Could you check a few things on this model? Use its own coordinates, in mm. A direction names the side the tool comes from. Coordinates: 2 decimals unless noted, no trailing zeros. Write each loop counter-clockwise with the first axis right and the second up, starting at its lowest first coordinate (ties: lowest second). Pieces come first, ordered by that corner, then holes.
```python
from build123d import *

# Parameters (mm, degrees)
SKETCH1_R           = 1.5
SKETCH1_R_2         = 4.25
SKETCH1_R_3         = 5
SKETCH1_R_4         = 1
BOSS_EXTRUDE2_DEPTH = 5
SKETCH2_W           = 0.5
SKETCH2_H           = 37
BOSS_EXTRUDE3_DEPTH = 5
CUT_EXTRUDE1_DEPTH  = 10
BOSS_EXTRUDE4_DEPTH = 5
SKETCH5_R           = 1.6
CUT_EXTRUDE2_DEPTH  = 10
BOSS_EXTRUDE5_DEPTH = 5
SKETCH7_R           = 1
BOSS_EXTRUDE6_DEPTH = 5


with BuildPart() as part:
    # Sketch1 → Boss-Extrude2 (new body)
    with BuildSketch(Plane.XY):
        with BuildLine():
            Line((45.25091594, -25.207708346), (50.00091594, -20.457708346))
            Line((50.00091594, -20.457708346), (50.00091594, 24.688738263))
            Line((50.00091594, 24.688738263), (45.147362549, 29.542291654))
            Line((45.147362549, 29.542291654), (26.35446933, 29.542291654))
            Line((26.35446933, 29.542291654), (21.25091594, 24.438738263))
            Line((21.25091594, 24.438738263), (21.25091594, 18.042291654))
            Line((21.25091594, 18.042291654), (20.408095363, 18.042291654))
            Line((20.408095363, 18.042291654), (16.70086026, 18.042291654))
            ThreePointArc((16.70086026, 18.042291654), (12.892426636, 17.542145454), (9.3422674, 16.075624987))
            ThreePointArc((9.3422674, 16.075624987), (2.182128173, 13.100539865), (-5.49908406, 12.043324729))
            Line((-5.49908406, 12.043324729), (-5.49908406, 12.039085999))
            ThreePointArc((-5.49908406, 12.039085999), (-15.49908406, 2.292291654), (-5.49908406, -7.454502691))
            Line((-5.49908406, -7.454502691), (-5.49908406, -7.458741422))
            ThreePointArc((-5.49908406, -7.458741422), (2.182128173, -8.515956557), (9.3422674, -11.491041679))
            ThreePointArc((9.3422674, -11.491041679), (12.892426636, -12.957562146), (16.70086026, -13.457708346))
            Line((16.70086026, -13.457708346), (20.408095363, -13.457708346))
            Line((20.408095363, -13.457708346), (21.25091594, -13.457708346))
            Line((21.25091594, -13.457708346), (21.25091594, -20.207708346))
            Line((21.25091594, -20.207708346), (26.25091594, -25.207708346))
            Line((26.25091594, -25.207708346), (45.25091594, -25.207708346))
        make_face()
        with Locations((46.75091594, -7.707708346)):
            Circle(SKETCH1_R, mode=Mode.SUBTRACT)
        with Locations((46.75091594, 12.292291654)):
            Circle(SKETCH1_R, mode=Mode.SUBTRACT)
        with Locations((33.50091594, 14.792291654)):
            Circle(SKETCH1_R_2, mode=Mode.SUBTRACT)
        with Locations((33.50091594, -10.207708346)):
            Circle(SKETCH1_R_2, mode=Mode.SUBTRACT)
        with Locations((19.25091594, 12.292291654)):
            Circle(SKETCH1_R, mode=Mode.SUBTRACT)
        with Locations((19.25091594, -7.707708346)):
            Circle(SKETCH1_R, mode=Mode.SUBTRACT)
        with Locations((-5.74908406, 2.292291654)):
            Circle(SKETCH1_R_3, mode=Mode.SUBTRACT)
        with Locations((1.25091594, 2.354746229)):
            Circle(SKETCH1_R_4, mode=Mode.SUBTRACT)
        with Locations((-5.686629485, -4.707708346)):
            Circle(SKETCH1_R_4, mode=Mode.SUBTRACT)
        with Locations((-12.74908406, 2.229837079)):
            Circle(SKETCH1_R_4, mode=Mode.SUBTRACT)
        with Locations((-5.811538636, 9.292291654)):
            Circle(SKETCH1_R_4, mode=Mode.SUBTRACT)
    extrude(amount=BOSS_EXTRUDE2_DEPTH)

    # Sketch2 → Boss-Extrude3 (add)
    with BuildSketch(Plane(origin=(0, 0, 0), x_dir=(-1, 0, 0), z_dir=(0, 0, -1))):
        Polygon((-26.25091594, -25.207708346), (-21.50091594, -25.207708346), (-21.50091594, -20.457708346), align=None)
        Polygon((-45.25091594, -25.207708346), (-45.50091594, -25.207708346), (-45.50091594, -24.957708346), align=None)
        Polygon((-45.50091594, 29.188738263), (-45.50091594, 29.792291654), (-21.50091594, 29.792291654), (-21.50091594, 24.688738263), (-26.35446933, 29.542291654), (-45.147362549, 29.542291654), align=None)
        with Locations((-50.25091594, 2.292291654)):
            Rectangle(SKETCH2_W, SKETCH2_H)
    extrude(amount=-BOSS_EXTRUDE3_DEPTH)

    # Sketch3 → Cut-Extrude1 (cut)
    with BuildSketch(Plane(origin=(0, 0, 0), x_dir=(-1, 0, 0), z_dir=(0, 0, -1))):
        Polygon((-50.00091594, -16.207708346), (-45.50091594, -16.207708346), (-45.50091594, -25.207708346), (-50.00091594, -20.457708346), align=None)
        Polygon((-50.50091594, 20.792291654), (-45.50091594, 20.792291654), (-45.50091594, 29.188738263), (-50.00091594, 24.688738263), align=None)
        Polygon((-21.50091594, -16.207708346), (-21.50091594, -20.457708346), (-21.25091594, -20.207708346), (-21.25091594, -16.207708346), align=None)
        Polygon((-21.50091594, 20.792291654), (-21.25091594, 20.792291654), (-21.25091594, 24.438738263), (-21.50091594, 24.688738263), align=None)
    extrude(amount=-CUT_EXTRUDE1_DEPTH, mode=Mode.SUBTRACT)

    # Sketch4 → Boss-Extrude4 (add)
    with BuildSketch(Plane(origin=(0, 0, 0), x_dir=(-1, 0, 0), z_dir=(0, 0, -1))):
        with BuildLine():
            Line((-21.25091594, 20.792291654), (-16.50091594, 20.792291654))
            Line((-16.50091594, 20.792291654), (-16.50091594, 18.040936414))
            ThreePointArc((-16.50091594, 18.040936414), (-16.600885803, 18.04195284), (-16.70086026, 18.042291654))
            Line((-16.70086026, 18.042291654), (-21.25091594, 18.042291654))
            Line((-21.25091594, 18.042291654), (-21.25091594, 20.792291654))
        make_face()
        with BuildLine():
            Line((-16.50091594, -13.456353106), (-16.50091594, -16.207708346))
            Line((-16.50091594, -16.207708346), (-21.25091594, -16.207708346))
            Line((-21.25091594, -16.207708346), (-21.25091594, -13.457708346))
            Line((-21.25091594, -13.457708346), (-16.70086026, -13.457708346))
            ThreePointArc((-16.70086026, -13.457708346), (-16.600885803, -13.457369532), (-16.50091594, -13.456353106))
        make_face()
    extrude(amount=-BOSS_EXTRUDE4_DEPTH)

    # Sketch5 → Cut-Extrude2 (cut)
    with BuildSketch(Plane.XY.offset(5)):
        with Locations((20.50091594, -7.707708346)):
            Circle(SKETCH5_R)
        with Locations((20.50091594, 12.292291654)):
            Circle(SKETCH5_R)
    extrude(amount=-CUT_EXTRUDE2_DEPTH, mode=Mode.SUBTRACT)

    # Sketch6 → Boss-Extrude5 (add)
    with BuildSketch(Plane.XY.offset(5)):
        with BuildLine():
            ThreePointArc((19.75191594, -6.293848735), (18.90091594, -7.707708346), (19.75191594, -9.121567957))
            ThreePointArc((19.75191594, -9.121567957), (17.75091594, -7.707708346), (19.75191594, -6.293848735))
        make_face()
        with BuildLine():
            ThreePointArc((19.75191594, 13.706151265), (18.90091594, 12.292291654), (19.75191594, 10.878432043))
            ThreePointArc((19.75191594, 10.878432043), (17.75091594, 12.292291654), (19.75191594, 13.706151265))
        make_face()
    extrude(amount=-BOSS_EXTRUDE5_DEPTH)

    # Sketch7 → Boss-Extrude6 (add)
    with BuildSketch(Plane(origin=(0, 0, 0), x_dir=(-1, 0, 0), z_dir=(0, 0, -1))):
        with Locations((-1.25091594, 2.354746229)):
            Circle(SKETCH7_R)
        with Locations((12.74908406, 2.229837079)):
            Circle(SKETCH7_R)
    extrude(amount=-BOSS_EXTRUDE6_DEPTH)


solid = part.part
```
1. For pin 1 (1 mm diameter, centred on x = 16.5, z = 1, fed in from +Y); pin 2 (7.5 mm diameter, centred on x = 33.5, y = -10.21, fed in from +Z); pin 3 (1 mm diameter, centred on y = 24, z = 0.5, fed in from -X); pin 4 (1.5 mm diameter, centred on x = 19, z = 2.5, fed in from -Y), each with a flat end and sliding along its axis, tell me the tip position at first contact or that it passes through.
Verdict:
pin 1: stops at y = 20.79
pin 2: passes through
pin 3: stops at x = 21.5
pin 4: stops at y = -16.21
2. I want a section at B-B on y = 6. Please give me the cut outline in (x, z), plus the area to 3 significant figures.
Verdict:
outline: (-14.77, 0) - (-9.1, 0) - (-9.1, 5) - (-14.77, 5) - close; (-2.39, 0) - (50.5, 0) - (50.5, 5) - (-2.39, 5) - close
area: 293 mm2
3. I want a section at A-A on x = -9.5. Please give me the cut outline in (y, z), plus the area to 3 significant figures.
Verdict:
outline: (-6.71, 0) - (-1.01, 0) - (-1.01, 5) - (-6.71, 5) - close; (5.6, 0) - (11.29, 0) - (11.29, 5) - (5.6, 5) - close
area: 56.9 mm2
4. If we mould it in two halves opening along Y, with no side actions, what happens to faces 5 (the face through (48, -16.208, 2)), 6 (the face through (45.501, -21, 2)), 7 (the face through (12.85, 17.53, 2.46)), 8 (the face through (-0.98, 3.79, 2.46))? For each: pulls with the +Y half, pulls with the -Y half, needs draft (parallel to the pull), parting line crosses it, or undercut.
Verdict:
face 5: pulls with the -Y half
face 6: needs draft
face 7: pulls with the +Y half
face 8: undercut
5. Please list where these lines run through material, in increasing order: line 1 along Y through (x, z) = (20, 0.9); line 2 along X through (y, z) = (20, 2.95); line 3 along X through (y, z) = (-19, 0.7).
Verdict:
line 1: y = -16.21 to -9.23, -6.19 to 10.77, 13.81 to 20.79
line 2: x = 16.5 to 50.5
line 3: x = 21.5 to 45.5
6. I want a section at D-D on y = 20. Please give me the cut outline in (x, z).
Verdict:
outline: (16.5, 0) - (50.5, 0) - (50.5, 5) - (16.5, 5) - close
7. I want a section at C-C on z = 2.5. Give the number of separate pieces and of enclosed holes in the cut face, plus the area to 3 significant figures.
Verdict:
separate pieces: 1
enclosed holes: 9
area: 2,160 mm2
8. On a 3-axis mill with a long thin cutter (end or side, diameter ignored), from which of +Z, -Z, +X, -X, +Y, -Y can I reach the whole of each face in a straight line? I mean faces 1 (the face through (45.501, 25, 2)), 2 (the face through (19, -16.208, 2)), 3 (the face through (19, 20.792, 2)), 4 (the face through (25, 3, 0)). Say none if no direction works.
Verdict:
face 1: +Z, -Z, +X, +Y
face 2: +Z, -Z, -X, -Y
face 3: +Z, -Z, -X, +Y
face 4: -Z, +X, -X, +Y, -Y
